from build123d import *

# Parameters (mm, degrees)
F0_W     = 14.351
F0_H     = 2.54
F0_W_2   = 1.524
F0_H_2   = 2.2225
F1_DEPTH = 25.4
F3_DEPTH = 25.4


with BuildPart() as f1:
    # F0 (on Top) → F1 (new body)
    with BuildSketch(Plane.XY):
        with Locations((7.1755, -1.27)):
            Rectangle(F0_W, F0_H)
        with Locations((15.113, -1.27)):
            Rectangle(F0_W_2, F0_H)
        with Locations((15.113, -3.65125)):
            Rectangle(F0_W_2, F0_H_2)
        with BuildLine():
            Line((15.875, -4.7625), (14.351, -4.7625))
            ThreePointArc((14.351, -4.7625), (20.6375, -11.049), (26.924, -4.7625))
            Line((26.924, -4.7625), (25.4, -4.7625))
            ThreePointArc((25.4, -4.7625), (20.6375, -9.525), (15.875, -4.7625))
        make_face()
    extrude(amount=F1_DEPTH)

    # F2 (on face) → F3 (cut)
    with BuildSketch(Plane.XZ.offset(2.54)):
        with BuildLine():
            ThreePointArc((8.73125, 12.7), (6.35, 15.08125), (3.96875, 12.7))
            ThreePointArc((3.96875, 12.7), (6.35, 10.31875), (8.73125, 12.7))
        make_face()
    extrude(amount=-F3_DEPTH, mode=Mode.SUBTRACT)


solid = f1.part
The listing builds one solid part. Answer for the finished solid, in the listing's coordinates (mm). A direction names the side the tool comes from. Give positions to 0.01 mm unless a question says otherwise; leave off trailing zeros. Write each loop counter-clockwise with the first axis right and the second up, starting at its lowest first coordinate (ties: lowest second). Pieces come first, ordered by that corner, then holes.
1) Section A-A (z = 12.7) is taken. Write down the section's boundary in (x, y) (1 decimal), and give its area (3 significant figures).
2) Section D-D (z = 5.25) is taken. Write down the section's boundary in (x, y) (1 decimal), and give its area (3 significant figures).
3) Section C-C (y = -7.5) is taken. Write down the section's boundary in (x, z), and give its area (3 significant figures).
4) Section B-B (x = 6.35) is taken. Write down the section's boundary in (y, z).
5) Given P1, Ø6, axis at x = 6.35, z = 12.7, coming from the -Y side; P2, Ø2, axis at x = 22.5, y = -7, coming from the +Z side; P3, Ø3, axis at y = -6.5, z = 5.5, coming from the -X side; P4, Ø6, axis at x = 17, y = -9, coming from the -Z side, each flat-ended and moving along its own axis, determine where each tip first touches the part or whether it passes through.
6) For a pull along X with two mould halves and no side action, classify faces 4 (the face through (20.499, -11.047, 12.522)), 5 (the face through (14, -2, 25.4)), 6 (the face through (14.351, -4, 13)), 7 (the face through (6.66, -1.29, 10.34)) as pulls with the +X half, pulls with the -X half, needs draft (parallel to the pull), parting line crosses it, or undercut.
7) A tool of negligible diameter and unlimited length cuts with its end or side. For faces 1 (the face through (15.875, -2, 13)), 2 (the face through (7.1, -2.54, 15.3)), 3 (the face through (10, 0, 13)), from which of +Z, -Z, +X, -X, +Y, -Y can it reach the whole face along a straight path? Write none if from no direction.
8) Find the intervals of material crossed by L1, parallel to X at y = -1.1, z = 12.7 (3 decimals); L2, parallel to Z at x = 6.35, y = -2; L3, parallel to Y at x = 3, z = 22.5, in increasing order.
Response:
1. outline: (0, -2.5) - (4, -2.5) - (4, 0) - (0, 0) - close; (8.7, -2.5) - (14.4, -2.5) - (14.4, -4.8) arc R6.3 ccw to (26.9, -4.8) - (25.4, -4.8) arc R4.8 cw to (15.9, -4.8) - (15.9, 0) - (8.7, 0) - close
1. area: 58.1 mm2
2. outline: (0, -2.5) - (14.4, -2.5) - (14.4, -4.8) arc R6.3 ccw to (26.9, -4.8) - (25.4, -4.8) arc R4.8 cw to (15.9, -4.8) - (15.9, 0) - (0, 0) - close
2. area: 70.2 mm2
3. outline: (14.98, 0) - (16.74, 0) - (16.74, 25.4) - (14.98, 25.4) - close; (24.53, 0) - (26.3, 0) - (26.3, 25.4) - (24.53, 25.4) - close
3. area: 89.5 mm2
4. outline: (-2.54, 0) - (0, 0) - (0, 10.32) - (-2.54, 10.32) - close; (-2.54, 15.08) - (0, 15.08) - (0, 25.4) - (-2.54, 25.4) - close
5. P1: stops at y = -2.54
5. P2: passes through
5. P3: stops at x = 14.36
5. P4: stops at z = 0
6. face 4: parting line crosses it
6. face 5: needs draft
6. face 6: pulls with the -X half
6. face 7: undercut
7. face 1: +Z, -Z, +X, +Y
7. face 2: +Z, -Z, -X, -Y
7. face 3: +Z, -Z, +X, -X, +Y
8. L1: x = 0 to 3.969, 8.731 to 15.875
8. L2: z = 0 to 10.32, 15.08 to 25.4
8. L3: y = -2.54 to 0
